Can you work these out from the model? Positions are in its coordinate system, mm. Face numbers are marked on the shaded views. A direction names the side the tool comes from. Give positions to 0.01 mm unless a question says otherwise; leave off trailing zeros. Order: outer loops, then holes, each group sorted by start corner. A loop starts at its lowest first (then second) coordinate and runs counter-clockwise, first axis right, second up.
Item 1: I'm going to push flat-ended pins straight in: pin 1 Ø4 at (x, y) = (19.05, 165.1) entering from -Z; pin 2 Ø9 at (x, y) = (6.35, 133.35) entering from -Z. Where does each tip first touch, or does it pass through?
Item 2: I want a section at D-D, the plane y = 94.5. Write out the boundary of the cut face in (x, z).
Item 3: I want a section at A-A, the plane z = -7.5. Write out the boundary of the cut face in (x, y), then the cut area to 3 significant figures.
Item 4: I want a section at C-C, the plane z = -31. Write out the boundary of the cut face in (x, y), then the cut area to 3 significant figures.
Item 5: I want a section at B-B, the plane x = 12.7. Write out the boundary of the cut face in (y, z), then the cut area to 3 significant figures.
Item 6: If I drill on line 1 along Y through (x, z) = (1.3, -38.1); line 2 along Y through (x, z) = (12.7, -1.2); line 3 along Z through (x, y) = (0.7, 165.1), over which ranges is the centre line in solid material (lowest first)?
Item 7: If we mould it in two halves opening along X, with no side actions, what happens to the marked faces 3, 4 and 5? For each: +X half, -X half, draft (parallel to the pull), parting line (faces both ways), or undercut.
Item 8: Which directions (+Z, -Z, +X, -X, +Y, -Y) give clear straight access to the entire face, cutting with the end or side of a thin tool? Please do the marked faces 1 and 2.
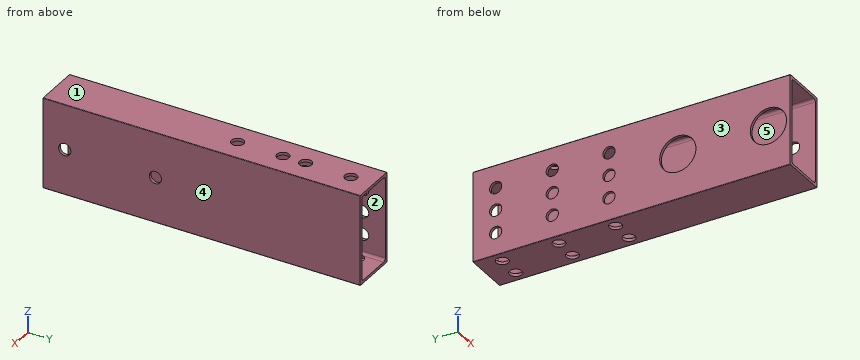
```python
from build123d import *

# Parameters (mm, degrees)
BOSS_EXTRUDE1_DEPTH = 177.8
SKETCH2_R           = 10.16
SKETCH2_R_2         = 3.429
CUT_EXTRUDE1_DEPTH  = 12.7
SKETCH2_3_R         = 3.429
CUT_EXTRUDE2_DEPTH  = 26.4
CUT_EXTRUDE3_START  = -1.5875
SKETCH3_R           = 3.429
CUT_EXTRUDE3_DEPTH  = 50.2125
SKETCH4_R           = 3.429
CUT_EXTRUDE4_DEPTH  = 2.54


with BuildPart() as part:
    # Sketch1 → Boss-Extrude1 (new body)
    with BuildSketch(Plane(origin=(0, 0, 0), x_dir=(1, 0, 0), z_dir=(0, 1, 0))):
        with BuildLine():
            Line((0.254, 50.8), (25.146, 50.8))
            ThreePointArc((25.146, 50.8), (25.325605122, 50.725605122), (25.4, 50.546))
            Line((25.4, 50.546), (25.4, 0.254))
            ThreePointArc((25.4, 0.254), (25.325605122, 0.074394878), (25.146, 0))
            Line((25.146, 0), (0.254, 0))
            ThreePointArc((0.254, 0), (0.074394878, 0.074394878), (0, 0.254))
            Line((0, 0.254), (0, 50.546))
            ThreePointArc((0, 50.546), (0.074394878, 50.725605122), (0.254, 50.8))
        make_face()
        with BuildLine():
            Line((1.5875, 3.1115), (1.5875, 47.6885))
            ThreePointArc((1.5875, 47.6885), (2.033869265, 48.766130735), (3.1115, 49.2125))
            Line((3.1115, 49.2125), (22.2885, 49.2125))
            ThreePointArc((22.2885, 49.2125), (23.366130735, 48.766130735), (23.8125, 47.6885))
            Line((23.8125, 47.6885), (23.8125, 3.1115))
            ThreePointArc((23.8125, 3.1115), (23.366130735, 2.033869265), (22.2885, 1.5875))
            Line((22.2885, 1.5875), (3.1115, 1.5875))
            ThreePointArc((3.1115, 1.5875), (2.033869265, 2.033869265), (1.5875, 3.1115))
        make_face(mode=Mode.SUBTRACT)
    extrude(amount=BOSS_EXTRUDE1_DEPTH)

    # Sketch2 → Cut-Extrude1 (cut)
    with BuildSketch(Plane.ZY):
        with Locations((-25.4, 12.192)):
            Circle(SKETCH2_R)
        with Locations((-25.4, 12.192)):
            Circle(SKETCH2_R_2, mode=Mode.SUBTRACT)
        with Locations((-25.4, 62.992)):
            Circle(SKETCH2_R)
        with Locations((-25.4, 62.992)):
            Circle(SKETCH2_R_2, mode=Mode.SUBTRACT)
        with Locations((-38.1, 165.1)):
            Circle(SKETCH2_R_2)
        with Locations((-25.4, 165.1)):
            Circle(SKETCH2_R_2)
        with Locations((-12.7, 165.1)):
            Circle(SKETCH2_R_2)
        with Locations((-25.4, 133.35)):
            Circle(SKETCH2_R_2)
        with Locations((-12.7, 133.35)):
            Circle(SKETCH2_R_2)
        with Locations((-25.4, 101.6)):
            Circle(SKETCH2_R_2)
        with Locations((-12.7, 101.6)):
            Circle(SKETCH2_R_2)
        with Locations((-38.1, 133.35)):
            Circle(SKETCH2_R_2)
        with Locations((-38.1, 101.6)):
            Circle(SKETCH2_R_2)
    extrude(amount=-CUT_EXTRUDE1_DEPTH, mode=Mode.SUBTRACT)

    # Sketch2<3> → Cut-Extrude2 (cut, through all)
    with BuildSketch(Plane.ZY):
        with Locations((-25.4, 12.192)):
            Circle(SKETCH2_3_R)
        with Locations((-25.4, 62.992)):
            Circle(SKETCH2_3_R)
    extrude(amount=-CUT_EXTRUDE2_DEPTH, mode=Mode.SUBTRACT)

    # Sketch3 → Cut-Extrude3 (cut, through all)
    with BuildSketch(Plane.XY.offset(CUT_EXTRUDE3_START)):
        with Locations((19.05, 165.1)):
            Circle(SKETCH3_R)
        with Locations((6.35, 165.1)):
            Circle(SKETCH3_R)
        with Locations((6.35, 133.35)):
            Circle(SKETCH3_R)
        with Locations((6.35, 101.6)):
            Circle(SKETCH3_R)
        with Locations((19.05, 133.35)):
            Circle(SKETCH3_R)
        with Locations((19.05, 101.6)):
            Circle(SKETCH3_R)
    extrude(amount=-CUT_EXTRUDE3_DEPTH, mode=Mode.SUBTRACT)

    # Sketch4 → Cut-Extrude4 (cut)
    with BuildSketch(Plane.XY):
        with Locations((12.7, 165.1)):
            Circle(SKETCH4_R)
        with Locations((12.7, 139.7)):
            Circle(SKETCH4_R)
        with Locations((12.7, 101.6)):
            Circle(SKETCH4_R)
        with Locations((12.7, 127)):
            Circle(SKETCH4_R)
    extrude(amount=-CUT_EXTRUDE4_DEPTH, mode=Mode.SUBTRACT)


solid = part.part
```
Results list:
1. pin 1: stops at z = -1.59
1. pin 2: stops at z = -50.8
2. outline: (0, -50.55) arc R0.25 ccw to (0.25, -50.8) - (25.15, -50.8) arc R0.25 ccw to (25.4, -50.55) - (25.4, -0.25) arc R0.25 ccw to (25.15, 0) - (0.25, 0) arc R0.25 ccw to (0, -0.25) - close; hole (1.59, -47.69) arc R1.52 ccw to (3.11, -49.21) - (22.29, -49.21) arc R1.52 ccw to (23.81, -47.69) - (23.81, -3.11) arc R1.52 ccw to (22.29, -1.59) - (3.11, -1.59) arc R1.52 ccw to (1.59, -3.11) - close
3. outline: (0, 0) - (1.59, 0) - (1.59, 177.8) - (0, 177.8) - close; (23.81, 0) - (25.4, 0) - (25.4, 177.8) - (23.81, 177.8) - close
3. area: 565 mm2
4. outline: (0, 0) - (1.59, 0) - (1.59, 3.71) - (0, 3.71) - close; (0, 20.67) - (1.59, 20.67) - (1.59, 54.51) - (0, 54.51) - close; (0, 71.47) - (1.59, 71.47) - (1.59, 177.8) - (0, 177.8) - close; (23.81, 0) - (25.4, 0) - (25.4, 177.8) - (23.81, 177.8) - close
4. area: 511 mm2
5. outline: (0, -50.8) - (177.8, -50.8) - (177.8, -49.21) - (0, -49.21) - close; (0, -1.59) - (98.17, -1.59) - (98.17, 0) - (0, 0) - close; (105.03, -1.59) - (123.57, -1.59) - (123.57, 0) - (105.03, 0) - close; (130.43, -1.59) - (136.27, -1.59) - (136.27, 0) - (130.43, 0) - close; (143.13, -1.59) - (161.67, -1.59) - (161.67, 0) - (143.13, 0) - close; (168.53, -1.59) - (177.8, -1.59) - (177.8, 0) - (168.53, 0) - close
5. area: 521 mm2
6. line 1: y = 0 to 98.17, 105.03 to 129.92, 136.78 to 161.67, 168.53 to 177.8
6. line 2: y = 0 to 98.17, 105.03 to 123.57, 130.43 to 136.27, 143.13 to 161.67, 168.53 to 177.8
6. line 3: z = -50.8 to -41.53, -34.67 to -28.83, -21.97 to -16.13, -9.27 to 0
7. face 3: -X half
7. face 4: +X half
7. face 5: undercut
8. face 1: +Z, +X, -X, +Y, -Y
8. face 2: +Y, -Y
